Source: three-view drawing plus pictorial views. Frame: mm from the lowest corner of the part. Coordinates: 2 decimals unless noted, no trailing zeros. Write each loop counter-clockwise with the first axis right and the second up, starting at its lowest first coordinate (ties: lowest second). Pieces come first, ordered by that corner, then holes. Notation, with made-up numbers: (-13, 48.5) - (22, 48.5) arc R9 ccw to (22, 52.5) - close; hole circle Ø7 at (-36, -7). An arc over 180 degrees is marked (long way). Put each result on its own line as item: value. Start each with the question number.
1. Cut plane B-B, the plane y = 8. Return loops of the section in (x, z) (1 decimal).
2. Cut plane C-C, the plane x = 100. Return loops of the section in (y, z), and give its area (3 significant figures).
3. Pin query (flat end, axial travel): pin 1 (2 mm diameter, centred on y = 31.5, z = 152.5, fed in from +X); pin 2 (3 mm diameter, centred on x = 81, z = 144.5, fed in from +Y); pin 3 (2.5 mm diameter, centred on x = 101.5, z = 101.5, fed in from +Y). Return the tip coordinate at first contact, or that it passes through.
4. Cut plane A-A, the plane z = 100. Return loops of the section in (x, y), and give its area (3 significant figures).
5. Line query: line 1 (X direction, y = 13, z = 100); line 2 (X direction, y = 18, z = 100); line 3 (X direction, y = 33.25, z = 100). Output: solid intervals per line, ascending.
6. Cut plane D-D, the plane y = 31.5. Return loops of the section in (x, z).
7. Pull-direction query (X, two-part tool) for the marked faces 1, 2 and 3; classes: released by +X, released by -X, zero draft, split by the parting line, or undercut.
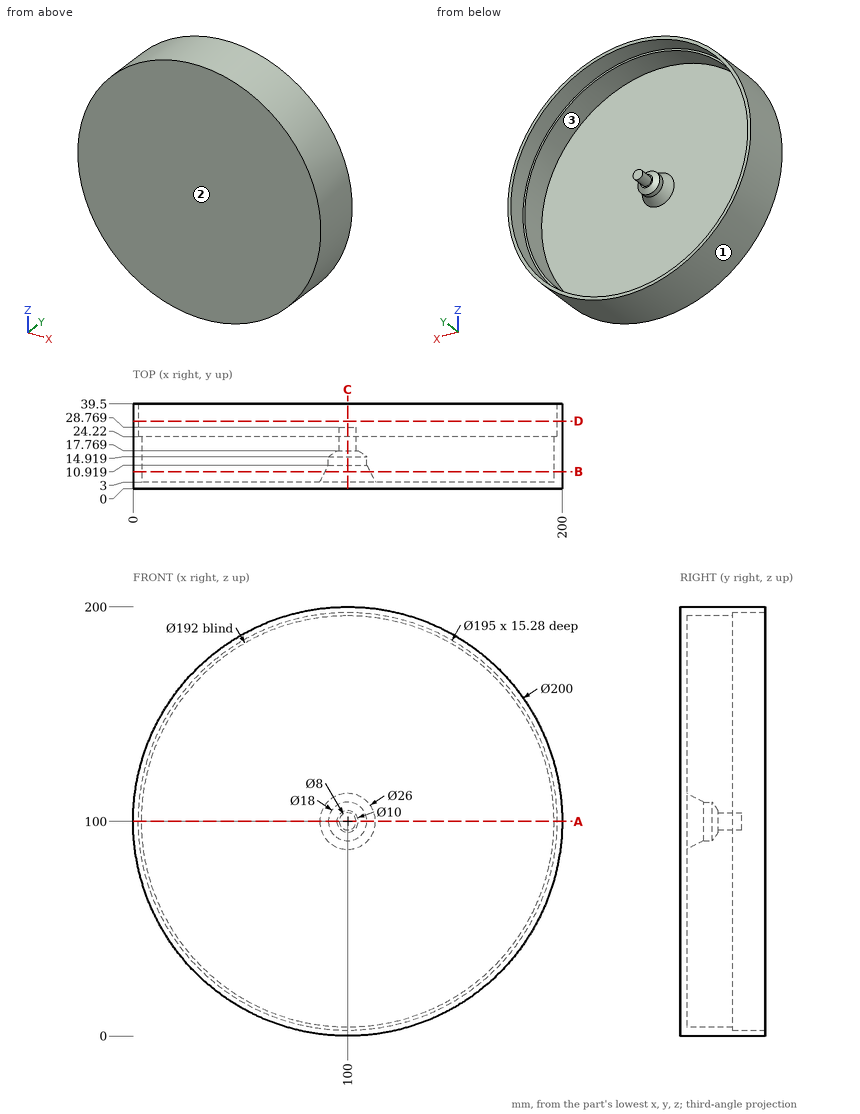
Report:
1. outline: circle Ø200 at (100, 100); circle Ø20.9 at (100, 100); hole circle Ø192 at (100, 100)
2. outline: (0, 0) - (39.5, 0) - (39.5, 2.5) - (24.22, 2.5) - (24.22, 4) - (3, 4) - (3, 87) - (10.92, 91) - (14.92, 91) - (17.77, 95) - (17.77, 96) - (28.77, 96) - (28.77, 104) - (17.77, 104) - (17.77, 105) - (14.92, 109) - (10.92, 109) - (3, 113) - (3, 196) - (24.22, 196) - (24.22, 197.5) - (39.5, 197.5) - (39.5, 200) - (0, 200) - close
2. area: 1,220 mm^2
3. pin 1: stops at x = 185.72
3. pin 2: stops at y = 3
3. pin 3: stops at y = 28.77
4. outline: (0, 0) - (200, 0) - (200, 39.5) - (197.5, 39.5) - (197.5, 24.22) - (196, 24.22) - (196, 3) - (113, 3) - (109, 10.92) - (109, 14.92) - (105, 17.77) - (104, 17.77) - (104, 28.77) - (96, 28.77) - (96, 17.77) - (95, 17.77) - (91, 14.92) - (91, 10.92) - (87, 3) - (4, 3) - (4, 24.22) - (2.5, 24.22) - (2.5, 39.5) - (0, 39.5) - close
4. area: 1,220 mm^2
5. line 1: x = 0 to 4, 91 to 109, 196 to 200
5. line 2: x = 0 to 4, 96 to 104, 196 to 200
5. line 3: x = 0 to 2.5, 197.5 to 200
6. outline: circle Ø200 at (100, 100); hole circle Ø195 at (100, 100)
7. face 1: split by the parting line
7. face 2: zero draft
7. face 3: undercut
